```python
from build123d import *

# Parameters (mm, degrees)
SWEEP1_PROFILE_R = 2.54


with BuildPart() as part:
    # Sweep1: sweep along a curve in space
    with BuildLine() as sweep1_path:
        Line((-119.38, 43.18, 0), (-75.65089034, 56.298732898, 0))
        ThreePointArc((-75.65089034, 56.298732898, 0), (-69.372940802, 56.156071327, 0), (-64.377963156, 52.350391225, 0))
        Line((-64.377963156, 52.350391225, 0), (-48.750110734, 29.776826615, 0))
        ThreePointArc((-48.750110734, 29.776826615, 0), (-45.111961937, 26.560482191, 0), (-40.396638066, 25.4, 0))
        Line((-40.396638066, 25.4, 0), (-10.16, 25.4, 0))
        ThreePointArc((-10.16, 25.4, 0), (-2.975795103, 22.424204897, 0), (0, 15.24, 0))
        Line((0, 15.24, 0), (0, 0, 0))
        Line((0, 0, 0), (0, -13.97, 0))
        ThreePointArc((0, -13.97, 0), (0, -17.562102448, 1.487897552), (0, -19.05, 5.08))
        Line((0, -19.05, 5.08), (0, -19.05, 16.427752875))
        ThreePointArc((0, -19.05, 16.427752875), (0, -16.47290998, 20.848368401), (0, -11.356361562, 20.783816937))
        Line((0, -11.356361562, 20.783816937), (0, 6.35, 10.16))
    # Sweep1 profile (on start of the path) → Sweep1 (sweep)
    with BuildSketch(Plane(origin=(-119.38, 43.18, 0), x_dir=(-0.2873478855663455, 0.9578262852211514, 0), z_dir=(0.9578262852211514, 0.2873478855663455, 0))):
        Circle(SWEEP1_PROFILE_R)
    sweep(path=sweep1_path.line)


solid = part.part
```
Design review of the part built by this model. Coordinates are the model's own, in mm. Coordinates: 2 decimals unless noted, no trailing zeros. Order: outer loops, then holes, each group sorted by start corner. A loop starts at its lowest first (then second) coordinate and runs counter-clockwise, first axis right, second up. Notation, with made-up numbers: M 14.5,87 L 53.5,87 A15 ccw 53.5,116 Z; hole C -31,80 d1. An arc over 180 degrees is marked long. Answer as a JSON object with one key per item and string values. Group by question number.
1) Wall thickness on L1, parallel to Z at x = -4, y = 22; L2, parallel to Z at x = -2.5, y = 18; L3, parallel to X at y = 7, z = 1.25: over which ranges is each line inside the solid? List them lowest first.
2) Add section B-B, the plane x = -16.5. Write out the cut boundary in (y, z).
3) Mouldability with a two-part tool opening along Z and no side actions: class faces 1 (the flat face through (0.04, 6.33, 10.13)), 2 (the flat face through (-119.37, 43.15, 0.04)), 3 (the cylindrical face through (-0.33, -16.53, 10.83)), 4 (the cylindrical face through (-25.067, 27.746, -0.973)) as pulls with the +Z half, pulls with the -Z half, needs draft (parallel to the pull), parting line crosses it, or undercut.
4) Add section A-A, the plane y = 14. Write out the cut boundary in (x, z).
5) For pin 1 (1.5 mm diameter, centred on x = -77, z = 0.5, fed in from -Y); pin 2 (3 mm diameter, centred on x = -24.5, z = 0, fed in from -Y), all flat-tipped, find the tip position at first contact; note any pin that passes through.
Computed values:
{
 "1": {"L1": "z = -2.33 to 2.33", "L2": "z = -1.54 to 1.54", "L3": "x = -2.21 to 2.21"},
 "2": {"outline": "C 25.4,0 d5.08"},
 "3": {"face 1": "undercut", "face 2": "needs draft", "face 3": "undercut", "face 4": "parting line crosses it"},
 "4": {"outline": "C 0,0 d5.08"},
 "5": {"pin 1": "stops at y = 53.04", "pin 2": "stops at y = 22.86"}
}
